from build123d import *

# Parameters (mm, degrees)
BOSS_EXTRUDE1_DEPTH = 5
CUT_EXTRUDE10_DEPTH = 7
SKETCH4_W           = 1.997648265
SKETCH4_H           = 6.998360209
CUT_EXTRUDE11_DEPTH = 1
SKETCH5_W           = 6
SKETCH5_H           = 3.997736752
CUT_EXTRUDE12_DEPTH = 3
CUT_EXTRUDE13_DEPTH = 3


with BuildPart() as part:
    # Sketch2 → Boss-Extrude1 (new body)
    with BuildSketch(Plane(origin=(0, 0, 0), x_dir=(1, 0, 0), z_dir=(0, 1, 0))):
        with BuildLine():
            Line((0, 3), (0, 3.998360209))
            Line((0, 3.998360209), (6, 3.998360209))
            Line((6, 3.998360209), (6, -3))
            Line((6, -3), (0, -3))
            ThreePointArc((0, -3), (-3, 0), (0, 3))
        make_face()
        with BuildLine():
            Line((0, 2), (2, 2))
            ThreePointArc((2, 2), (4, 0), (2, -2))
            Line((2, -2), (0, -2))
            ThreePointArc((0, -2), (-2, 0), (0, 2))
        make_face(mode=Mode.SUBTRACT)
    extrude(amount=BOSS_EXTRUDE1_DEPTH)

    # Sketch3 → Cut-Extrude10 (cut)
    with BuildSketch(Plane.XY.offset(3)):
        Polygon((3, 5), (-3, 5), (-3, 4), (-3, 2), (0, 2), (0, 4), (3, 4), align=None)
    extrude(amount=-CUT_EXTRUDE10_DEPTH, mode=Mode.SUBTRACT)

    # Sketch4 → Cut-Extrude11 (cut)
    with BuildSketch(Plane.XZ):
        with Locations((5.001175868, -0.499180105)):
            Rectangle(SKETCH4_W, SKETCH4_H)
    extrude(amount=-CUT_EXTRUDE11_DEPTH, mode=Mode.SUBTRACT)

    # Sketch5 → Cut-Extrude12 (cut)
    with BuildSketch(Plane.XZ):
        with Locations((3, 0.001131624)):
            Rectangle(SKETCH5_W, SKETCH5_H)
    extrude(amount=-CUT_EXTRUDE12_DEPTH, mode=Mode.SUBTRACT)

    # 3DSketch1 → Cut-Extrude13 (cut, along a direction that is not the sketch's normal)
    with BuildSketch(Plane(origin=(0, 2, 2), x_dir=(0.6666666666666625, 0.66666666666667, 0.3333333333333349), z_dir=(0.4472135954999618, 0, -0.894427190999914))):
        Polygon((0, 0), (1.333333333, -1.490711985), (3, 0), (1.661678745, 1.496288651), align=None)
    extrude(amount=-CUT_EXTRUDE13_DEPTH, dir=(0, 0, -1), mode=Mode.SUBTRACT)


solid = part.part
Design review of the part built by this model. Coordinates are the model's own, in mm. A direction names the side the tool comes from. Coordinates: 2 decimals unless noted, no trailing zeros. Write each loop counter-clockwise with the first axis right and the second up, starting at its lowest first coordinate (ties: lowest second). Pieces come first, ordered by that corner, then holes. Notation, with made-up numbers: (25, -22) - (30, -22) arc R15 ccw to (30, -9) - close; hole circle Ø2 at (45, 84.25). An arc over 180 degrees is marked (long way). One line per item, written item: value.
1) For faces 5 (the face through (0, 2.4, -3.2)), 6 (the face through (5, 1, 2.5)), 7 (the face through (1, 4, -3)), list the 3-axis set-ups (+Z, -Z, +X, -X, +Y, -Y) from which the entire face can be reached by the end or side of a thin tool; tool diameter is ignored.
Answer sheet:
face 5: -Z, -X, +Y
face 6: +Z, -Z, +X, -Y
face 7: +Z, -Z, -X, +Y
2) Mouldability with a two-part tool opening along Z and no side actions: class faces 1 (the face through (5, 3, 0)), 2 (the face through (3, 2, -3.998)), 3 (the face through (4, 4, 0)), 4 (the face through (4.002, 0.5, 2.5)) as +Z half, -Z half, draft (parallel to the pull), parting line (faces both ways), or undercut.
Answer sheet:
face 1: undercut
face 2: -Z half
face 3: undercut
face 4: draft
3) Add section C-C (y = 1.65). State the section outline as (x, z) points.
Answer sheet:
outline: (0, -4) - (6, -4) - (6, -2) - (2.1, -2) arc R2 cw to (2, -2) - (0, -2) arc R2 cw to (0, 2) - (6, 2) - (6, 3) - (0, 3) arc R3 ccw to (0, -3) - close
4) Add section A-A (z = 0). State the section outline as (x, y) points, plus the area to 3 significant figures.
Answer sheet:
outline: (-3, 0) - (-2, 0) - (-2, 2) - (-3, 2) - close; (4, 3) - (6, 3) - (6, 5) - (4, 5) - close
area: 6.00 mm2
5) Add section D-D (x = -1.5). State the section outline as (y, z) points.
Answer sheet:
outline: (0, -2.6) - (2, -2.6) - (2, -1.32) - (0, -1.32) - close; (0, 1.32) - (2, 1.32) - (2, 2.6) - (0, 2.6) - close
6) Insertion check: pin 1 (0.6 mm diameter, centred on x = 5, z = -3.5, fed in from -Y); pin 2 (1.1 mm diameter, centred on y = 0.5, z = -3, fed in from +X); pin 3 (1.5 mm diameter, centred on y = 1, z = -1, fed in from +X); pin 4 (2.5 mm diameter, centred on x = -1.5, z = 0, fed in from +Y). Each pin has a flat end and moves straight along its axis. Give the tip position at first contact, or say it passes through.
Answer sheet:
pin 1: stops at y = 1
pin 2: stops at x = 6
pin 3: stops at x = -0.97
pin 4: stops at y = 2
7) Add section B-B (x = 0.25). State the section outline as (y, z) points (3 decimals).
Answer sheet:
outline: (0, -3.998) - (4, -3.998) - (4, -2) - (0, -2) - close; (0, 2) - (4, 2) - (4, 2.125) - (1.999, 2.125) - (1.999, 3) - (0, 3) - close
8) To check wall thickness, follow probe 1 along Z at (x, y) = (4, 1); probe 2 along Y at (x, z) = (2.25, -2.5); probe 3 along Y at (x, z) = (5.75, 2.5). State the ranges of each line that lie inside material, in increasing order.
Answer sheet:
probe 1: z = -4 to -2, 2 to 3
probe 2: y = 0 to 4
probe 3: y = 1 to 5
